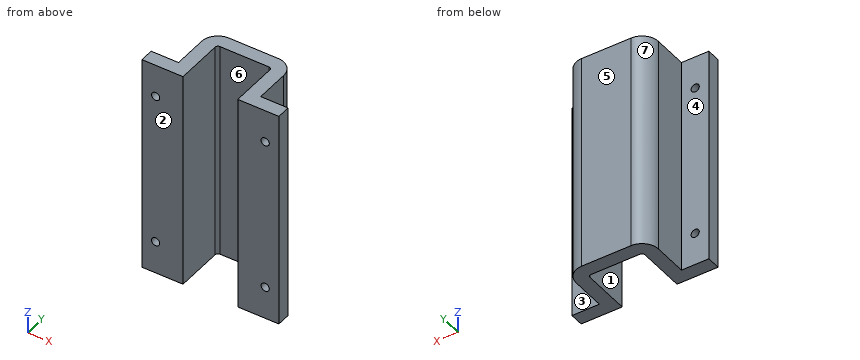
from build123d import *

# Parameters (mm, degrees)
BOSS_EXTRUDE1_DEPTH   = 80
F_3_0MM_DOWEL_HOLE1_D = 3


with BuildPart() as part:
    # Sketch1 → Boss-Extrude1 (new body)
    with BuildSketch(Plane.XY):
        with BuildLine():
            Line((9, 15), (-9, 15))
            ThreePointArc((-9, 15), (-13.242640687, 13.242640687), (-15, 9))
            Line((-15, 9), (-15, -3.5))
            Line((-15, -3.5), (-25, -3.5))
            Line((-25, -3.5), (-25, -8.5))
            Line((-25, -8.5), (-10, -8.5))
            Line((-10, -8.5), (-10, 9))
            ThreePointArc((-10, 9), (-9.707106781, 9.707106781), (-9, 10))
            Line((-9, 10), (9, 10))
            ThreePointArc((9, 10), (9.707106781, 9.707106781), (10, 9))
            Line((10, 9), (10, -8.5))
            Line((10, -8.5), (25, -8.5))
            Line((25, -8.5), (25, -3.5))
            Line((25, -3.5), (15, -3.5))
            Line((15, -3.5), (15, 9))
            ThreePointArc((15, 9), (13.242640687, 13.242640687), (9, 15))
        make_face()
    extrude(amount=BOSS_EXTRUDE1_DEPTH)

    # Ø3.0mm Dowel Hole1 (through all)
    with Locations(Plane(origin=(0, -3.5, 0), x_dir=(1, 0, 0), z_dir=(0, 1, 0))):
        with Locations((-20, -12), (-20, -68), (20, -12), (20, -68)):
            Hole(F_3_0MM_DOWEL_HOLE1_D / 2)


solid = part.part
Verification items for the finished model (mm, model axes). Face numbers are marked on the shaded views. A direction names the side the tool comes from. Give positions to 0.01 mm unless a question says otherwise; leave off trailing zeros. Write each loop counter-clockwise with the first axis right and the second up, starting at its lowest first coordinate (ties: lowest second). Pieces come first, ordered by that corner, then holes. Notation, with made-up numbers: M 82.25,33 L 99.25,33 A7 ccw 99.25,38 Z; hole C 69.5,19.25 d6. An arc over 180 degrees is marked long. Write item = value, one per line.
(1) Sectioned sample at A-A (y = -0.5). Record the cut outline in (x, z).
Found:
outline = M -15,0 L -10,0 L -10,80 L -15,80 Z; M 10,0 L 15,0 L 15,80 L 10,80 Z
(2) Sectioned sample at B-B (x = -20). Record the cut outline in (y, z), then the cut area to 3 significant figures.
Found:
outline = M -8.5,0 L -3.5,0 L -3.5,10.5 L -8.5,10.5 Z; M -8.5,13.5 L -3.5,13.5 L -3.5,66.5 L -8.5,66.5 Z; M -8.5,69.5 L -3.5,69.5 L -3.5,80 L -8.5,80 Z
area = 370 mm2
(3) Access from +Z, -Z, +X, -X, +Y, -Y to the whole of each face (thin tool, end or side, straight path). Record for the marked faces 1, 2, 3 and 4.
Found:
face_1 = +Z, -Z, -Y
face_2 = +Z, -Z, +X, -X, -Y
face_3 = +Z, -Z, +X, +Y
face_4 = +Z, -Z, -X, +Y
(4) Sectioned sample at D-D (z = 44.5). Record the cut outline in (x, y).
Found:
outline = M -25,-8.5 L -10,-8.5 L -10,9 A1 cw -9,10 L 9,10 A1 cw 10,9 L 10,-8.5 L 25,-8.5 L 25,-3.5 L 15,-3.5 L 15,9 A6 ccw 9,15 L -9,15 A6 ccw -15,9 L -15,-3.5 L -25,-3.5 Z
(5) Material ranges on line 1 (X direction, y = -6.65, z = 68); line 2 (Z direction, x = 20, y = -5.7); line 3 (X direction, y = -5, z = 53.5), recorded low to high.
Found:
line_1 = -25 to -21.5, -18.5 to -10, 10 to 18.5, 21.5 to 25
line_2 = 0 to 10.5, 13.5 to 66.5, 69.5 to 80
line_3 = -25 to -10, 10 to 25
(6) Draft check along X on the marked faces 5, 6 and 7. Enter one of: released by +X, released by -X, zero draft, split by the parting line, or undercut.
Found:
face_5 = zero draft
face_6 = undercut
face_7 = released by -X
(7) Sectioned sample at C-C (z = 68). Record the cut outline in (x, y), then the cut area to 3 significant figures.
Found:
outline = M -25,-8.5 L -21.5,-8.5 L -21.5,-3.5 L -25,-3.5 Z; M -18.5,-8.5 L -10,-8.5 L -10,9 A1 cw -9,10 L 9,10 A1 cw 10,9 L 10,-8.5 L 18.5,-8.5 L 18.5,-3.5 L 15,-3.5 L 15,9 A6 ccw 9,15 L -9,15 A6 ccw -15,9 L -15,-3.5 L -18.5,-3.5 Z; M 21.5,-8.5 L 25,-8.5 L 25,-3.5 L 21.5,-3.5 Z
area = 390 mm2
(8) Go/stop test with flat-tipped pins: pin 1 Ø2 at (y, z) = (11, 21) entering from -X; pin 2 Ø1.8 at (x, z) = (20, 68) entering from +Y; pin 3 Ø5 at (y, z) = (0, 46.5) entering from +X; pin 4 Ø12 at (x, y) = (18, 3) entering from +Z. Record where each tip stops, or that it passes through.
Found:
pin_1 = -14.92
pin_2 = through
pin_3 = 15
pin_4 = 80
